Geometry: see drawing. Coordinates: mm, zero at the bounding-box minimum. A direction names the side the tool comes from. Coordinates: 2 decimals unless noted, no trailing zeros. Loops run counter-clockwise (first coordinate to the right, second up) from the corner with the lowest first, then second, coordinate; pieces in that order, holes last.
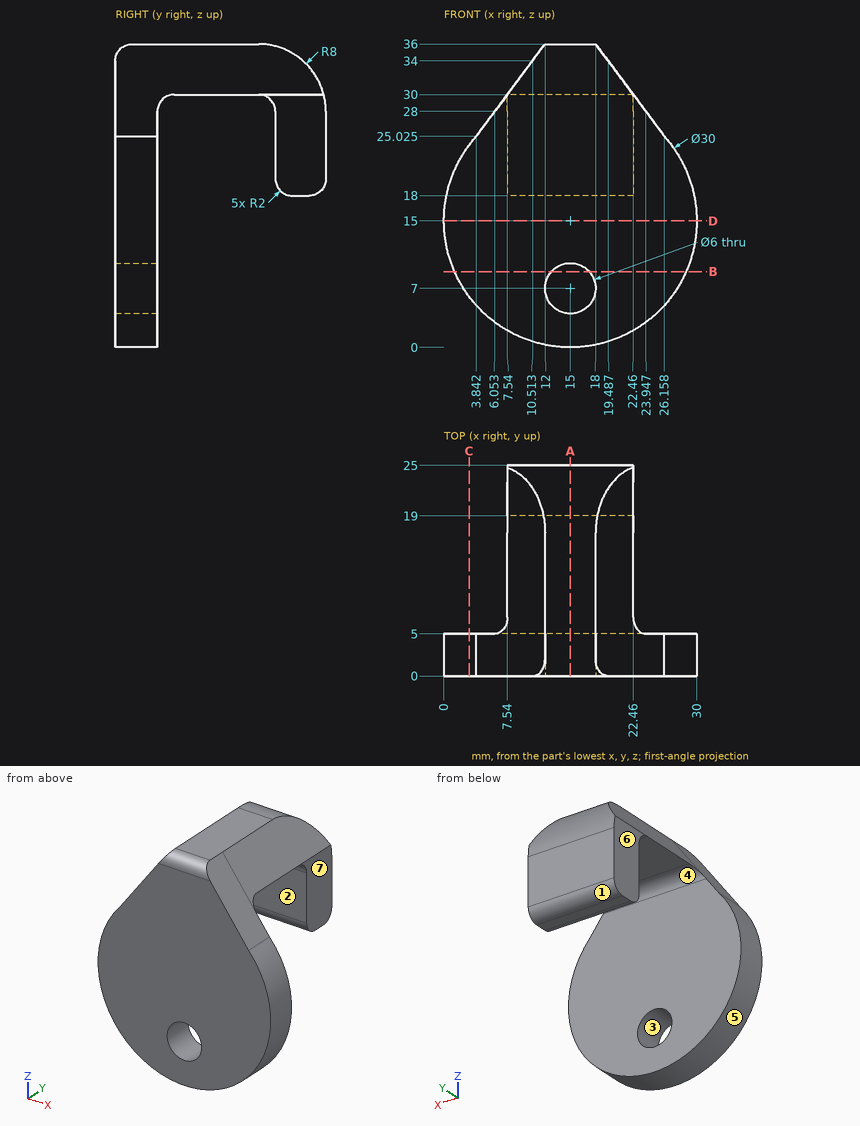
Item 1: Section query C-C (x = 3). Output: boundary loops of the cut face in (y, z), then the cut area to 3 significant figures.
Result:
outline: (0, 6) - (5, 6) - (5, 24) - (0, 24) - close
area: 90.0 mm2
Item 2: Reachability of the marked faces 4, 5, 6 and 7 from +Z, -Z, +X, -X, +Y, -Y: full face, straight path, thin tool, end or side. Return the list, or none.
Result:
face 4: -Z, +X, -X
face 5: +Y, -Y
face 6: +Z, -Z, -X, +Y
face 7: +Z, -Z, +X, +Y
Item 3: Section query D-D (z = 15). Output: boundary loops of the cut face in (x, y), then the cut area to 3 significant figures.
Result:
outline: (0, 0) - (30, 0) - (30, 5) - (0, 5) - close
area: 150 mm2
Item 4: Section query B-B (z = 9). Output: boundary loops of the cut face in (x, y), then the cut area to 3 significant figures.
Result:
outline: (1.25, 0) - (12.76, 0) - (12.76, 5) - (1.25, 5) - close; (17.24, 0) - (28.75, 0) - (28.75, 5) - (17.24, 5) - close
area: 115 mm2
Item 5: Line query: L1, parallel to Y at x = 15, z = 25; L2, parallel to Y at x = 24, z = 23.5; L3, parallel to Z at x = 12.5, y = 14.25. Output: solid intervals per line, ascending.
Result:
L1: y = 0 to 5, 19 to 25
L2: y = 0 to 5
L3: z = 30 to 36
Item 6: Contact query for flat-ended pins moving along their axis: P1, Ø10, axis at x = 6, y = 5, coming from the -Z side; P2, Ø2.5, axis at y = 19, z = 23, coming from the -X side; P3, Ø4, axis at y = 6, z = 21, coming from the -X side; P4, Ø5, axis at x = 15, z = 7, coming from the -Y side. Output: stop coordinate, or through.
Result:
P1: stops at z = 0.54
P2: stops at x = 7.54
P3: stops at x = 0.62
P4: passes through
Item 7: Section query A-A (x = 15). Output: boundary loops of the cut face in (y, z).
Result:
outline: (0, 0) - (5, 0) - (5, 4) - (0, 4) - close; (0, 10) - (5, 10) - (5, 28) arc R2 cw to (7, 30) - (17, 30) arc R2 cw to (19, 28) - (19, 20) arc R2 ccw to (21, 18) - (23, 18) arc R2 ccw to (25, 20) - (25, 28) arc R8 ccw to (17, 36) - (2, 36) arc R2 ccw to (0, 34) - close
Item 8: Mould query, pull axis Y, two halves, no side actions, for the marked faces 1, 2 and 3. Classes: +Y half, -Y half, draft (parallel to the pull), parting line (faces both ways), or undercut.
Result:
face 1: +Y half
face 2: undercut
face 3: draft
